Input: part model. Units: mm. Frame: model coordinates. Coordinates: 2 decimals unless noted, no trailing zeros. Loops run counter-clockwise (first coordinate to the right, second up) from the corner with the lowest first, then second, coordinate; pieces in that order, holes last. Notation, with made-up numbers: M 10.25,18 L 28.25,18 A36 cw 28.25,55 Z; hole C 20,32 d5. An arc over 180 degrees is marked long. Use a Markdown table: item, result. Add a question column.
1. Line query: L1, parallel to X at y = 3, z = 1; L2, parallel to Z at x = -10, y = 2; L3, parallel to Y at x = -7.75, z = 9.25. Output: solid intervals per line, ascending. Write a range as [from, to].
2. Draft query along Z for faces 1 (the cylindrical face through (0.37, 4.93, -8.34)), 2 (the cylindrical face through (-3.955, -24.65, -5.158)), 3 (the flat face through (-5, 0, 5)), 4 (the cylindrical face through (-8.5, 4.93, -0.07)). Return one class per face: +Z half, -Z half, draft (parallel to the pull), parting line (faces both ways), or undercut.
3. Section D-D on z = 10. Output: boundary loops of the cut face in (x, y).
4. Section C-C on y = 3.5. State how many separate pieces and enclosed holes the cut face has, then the cut area to 3 significant figures.
5. Section A-A on x = 0. Output: boundary loops of the cut face in (y, z).
6. Pin query (flat end, axial travel): pin 1 (4 mm diameter, centred on y = -37.5, z = -4.5, fed in from +X); pin 2 (4 mm diameter, centred on x = 8.66, z = 5, fed in from -Y); pin 3 (5 mm diameter, centred on y = -32, z = 3.5, fed in from +X). Return the tip coordinate at first contact, or that it passes through.
7. Section B-B on z = 0. Output: boundary loops of the cut face in (x, y).
```python
from build123d import *

# Parameters (mm, degrees)
SKETCH1_R             = 12.5
BOSS_EXTRUDE1_DEPTH   = 10
M3_CLEARANCE_HOLE1_D  = 3.4
F_3_0MM_DOWEL_HOLE1_D = 3
SKETCH7_R             = 6.5
BOSS_EXTRUDE2_DEPTH   = 50


with BuildPart() as part:
    # Sketch1 → Boss-Extrude1 (new body)
    with BuildSketch(Plane(origin=(0, 0, 0), x_dir=(1, 0, 0), z_dir=(0, 1, 0))):
        with Locations(Location((0, 0, 0), (0, 0, 270))):
            Circle(SKETCH1_R)
    extrude(amount=BOSS_EXTRUDE1_DEPTH)

    # M3 Clearance Hole1 (through all)
    with Locations(Plane(origin=(0, 10, 0), x_dir=(1, 0, 0), z_dir=(0, 1, 0))):
        with Locations((-8.660254038, 5), (0, 10), (8.660254038, 5), (8.660254038, -5), (0, -10), (-8.660254038, -5)):
            Hole(M3_CLEARANCE_HOLE1_D / 2)

    # Ø3.0mm Dowel Hole1 (through all)
    with Locations(Plane(origin=(0, 10, 0), x_dir=(1, 0, 0), z_dir=(0, 1, 0))):
        with Locations((-10, 0), (10, 0)):
            Hole(F_3_0MM_DOWEL_HOLE1_D / 2)

    # Sketch7 → Boss-Extrude2 (add)
    with BuildSketch(Plane(origin=(0, 0, 0), x_dir=(1, 0, 0), z_dir=(0, 1, 0))):
        with Locations(Location((0, 0, 0), (0, 0, 270))):
            Circle(SKETCH7_R)
    extrude(amount=-BOSS_EXTRUDE2_DEPTH)


solid = part.part
```
Answers below:
| question | item | result |
|---|---|---|
| 1 | L1 | x = [-12.46, -11.12], [-8.88, 8.88], [11.12, 12.46] |
| 1 | L2 | z = [-7.5, -6.05], [-3.95, -1.5], [1.5, 3.95], [6.05, 7.5] |
| 1 | L3 | y = [0, 10] |
| 2 | face 1 | undercut |
| 2 | face 2 | parting line |
| 2 | face 3 | draft |
| 2 | face 4 | undercut |
| 3 | outline | M -7.5,0 L -1.7,0 L -1.7,10 L -7.5,10 Z; M 1.7,0 L 7.5,0 L 7.5,10 L 1.7,10 Z |
| 4 | separate pieces | 1 |
| 4 | enclosed holes | 8 |
| 4 | area | 422 mm² |
| 5 | outline | M -50,-6.5 L 0,-6.5 L 0,-8.3 L 10,-8.3 L 10,8.3 L 0,8.3 L 0,6.5 L -50,6.5 Z; M 0,-12.5 L 10,-12.5 L 10,-11.7 L 0,-11.7 Z; M 0,11.7 L 10,11.7 L 10,12.5 L 0,12.5 Z |
| 6 | pin 1 | stops at x = 6 |
| 6 | pin 2 | stops at y = 0 |
| 6 | pin 3 | stops at x = 6.42 |
| 7 | outline | M -12.5,0 L -11.5,0 L -11.5,10 L -12.5,10 Z; M -8.5,0 L -6.5,0 L -6.5,-50 L 6.5,-50 L 6.5,0 L 8.5,0 L 8.5,10 L -8.5,10 Z; M 11.5,0 L 12.5,0 L 12.5,10 L 11.5,10 Z |
